Here's how the part is built. I have some questions about the finished solid (model axes, mm). A direction names the side the tool comes from. Coordinates: 2 decimals unless noted, no trailing zeros. Loops run counter-clockwise (first coordinate to the right, second up) from the corner with the lowest first, then second, coordinate; pieces in that order, holes last.
from build123d import *

# Parameters (mm, degrees)
CYLINDER098_R          = 1.8
CYLINDER098_DEPTH      = 5
ARRAY001_X_COUNT       = 2
ARRAY001_X_PITCH       = 31
ARRAY001_Y_COUNT       = 2
ARRAY001_Y_PITCH       = 31
CYLINDER_R             = 2.2
CYLINDER_DEPTH         = 20
ARRAY_X_COUNT          = 2
ARRAY_X_PITCH          = 30
ARRAY_Y_COUNT          = 2
ARRAY_Y_PITCH          = 20
ARRAY_PLACEMENT_ANGLE  = 90
CYLINDER097_R          = 11.5
CYLINDER097_DEPTH      = 5
BOX006_W               = 53
BOX006_H               = 5
BOX006_DEPTH           = 30
BOX005_W               = 53
BOX005_H               = 53
BOX005_DEPTH           = 5
FILLET001_R            = 10
PAD001_DEPTH           = 5
ARRAY002_X_COUNT       = 2
ARRAY002_X_PITCH       = 48
CUT004_ROLL_ANGLE      = 90
CUT004_PLACEMENT_ANGLE = -90


with BuildPart() as stepper_bolt_hole_array:
    # Cylinder098 → Cylinder098 (new body)
    with BuildSketch(Plane.XY):
        Circle(CYLINDER098_R)
    extrude(amount=CYLINDER098_DEPTH)

    # Array001 X: stepper bolt hole array ×2


with BuildPart() as stepper_bolt_hole_array_1:
    add(stepper_bolt_hole_array.part)
    with Locations(*[(i * ARRAY001_X_PITCH, 0, 0) for i in range(1, ARRAY001_X_COUNT)]):
        add(stepper_bolt_hole_array.part)

    # Array001 Y: stepper bolt hole array ×2


with BuildPart() as stepper_bolt_hole_array_2:
    add(stepper_bolt_hole_array_1.part)
    with Locations(*[(0, i * ARRAY001_Y_PITCH, 0) for i in range(1, ARRAY001_Y_COUNT)]):
        add(stepper_bolt_hole_array_1.part)


with BuildPart() as stepper_bolt_hole_array_3:
    # Array001 placement: moved
    add(stepper_bolt_hole_array_2.part.moved(Location((-15.5, -15.5, 0))))


with BuildPart() as insert_hole_array:
    # Cylinder → Cylinder (new body)
    with BuildSketch(Plane.XY.offset(-3)):
        Circle(CYLINDER_R)
    extrude(amount=CYLINDER_DEPTH)

    # Array X: insert hole array ×2


with BuildPart() as insert_hole_array_1:
    add(insert_hole_array.part)
    with Locations(*[(i * ARRAY_X_PITCH, 0, 0) for i in range(1, ARRAY_X_COUNT)]):
        add(insert_hole_array.part)

    # Array Y: insert hole array ×2


with BuildPart() as insert_hole_array_2:
    add(insert_hole_array_1.part)
    with Locations(*[(0, i * ARRAY_Y_PITCH, 0) for i in range(1, ARRAY_Y_COUNT)]):
        add(insert_hole_array_1.part)


with BuildPart() as insert_hole_array_3:
    # Array placement: moved
    add(insert_hole_array_2.part.moved(Location((-15, -20.5, 10))).rotate(Axis((-15, -20.5, 10), (1, 0, 0)), ARRAY_PLACEMENT_ANGLE))


with BuildPart() as stepper_mount_holes:
    # Cylinder097 → Cylinder097 (new body)
    with BuildSketch(Plane.XY):
        Circle(CYLINDER097_R)
    extrude(amount=CYLINDER097_DEPTH)

    # Fusion006: union stepper bolt hole array, insert hole array
    add(stepper_bolt_hole_array_3.part)
    add(insert_hole_array_3.part)


with BuildPart() as stepper_mount_bottom:
    # Box006 → Box006 (new body)
    with BuildSketch(Plane(origin=(-26.5, -26.5, 5), x_dir=(1, 0, 0), z_dir=(0, 0, 1))):
        with Locations((26.5, 2.5)):
            Rectangle(BOX006_W, BOX006_H)
    extrude(amount=BOX006_DEPTH)


with BuildPart() as stepper_mount_cube_fillet:
    # Box005 → Box005 (new body)
    with BuildSketch(Plane(origin=(-26.5, -26.5, 0), x_dir=(1, 0, 0), z_dir=(0, 0, 1))):
        with Locations((26.5, 26.5)):
            Rectangle(BOX005_W, BOX005_H)
    extrude(amount=BOX005_DEPTH)

    # Fillet001
    fillet001_edges = [stepper_mount_cube_fillet.edges().sort_by_distance(p)[0] for p in [
        (-26.5, 26.5, 2.5),
        (26.5, 26.5, 2.5),
    ]]
    fillet(fillet001_edges, radius=FILLET001_R)


with BuildPart() as stepper_mount_cut:
    # Sketch001 → Pad001 (new body)
    with BuildSketch(Plane.YZ):
        Polygon((-26.5, 5), (-3.224222, 5), (-26.5, 35), align=None)
    extrude(amount=PAD001_DEPTH)

    # Array002 X: stepper mount cut ×2


with BuildPart() as stepper_mount_cut_1:
    add(stepper_mount_cut.part)
    with Locations(*[(i * ARRAY002_X_PITCH, 0, 0) for i in range(1, ARRAY002_X_COUNT)]):
        add(stepper_mount_cut.part)


with BuildPart() as stepper_mount_cut_2:
    # Array002 placement: moved
    add(stepper_mount_cut_1.part.moved(Location((-26.5, 0, 0))))

    # Fusion007: union stepper mount bottom, stepper mount cube fillet
    add(stepper_mount_bottom.part)
    add(stepper_mount_cube_fillet.part)

    # Cut004: cut stepper mount holes
    add(stepper_mount_holes.part, mode=Mode.SUBTRACT)


with BuildPart() as stepper_mount_cut_3:
    # Cut004 roll: moved
    add(stepper_mount_cut_2.part.rotate(Axis((0, 0, 0), (1, 0, 0)), CUT004_ROLL_ANGLE))


with BuildPart() as stepper_mount_cut_4:
    # Cut004 placement: moved
    add(stepper_mount_cut_3.part.moved(Location((0, 0, 21.5))).rotate(Axis((0, 0, 21.5), (0, 0, 1)), CUT004_PLACEMENT_ANGLE))


solid = stepper_mount_cut_4.part
Q1. Will these pins go through, and if not, where does the flat tip stop? P1, Ø20.5, axis at y = 0, z = 21.5, coming from the -X side; P2, Ø2, axis at x = -29.5, y = -13.5, coming from the +Z side; P3, Ø8, axis at y = -3, z = 42.5, coming from the -X side.
Q2. We'd pull the mould along X, two halves only. Please class faces 1 (the cylindrical face through (-10.66, -17.1, -2.46)), 2 (the flat face through (-2, 0, 48)), 3 (the flat face through (-35, 0, -2)): pulls with the +X half, pulls with the -X half, needs draft (parallel to the pull), parting line crosses it, or undercut.
Q3. Suppose I cut it at B-B on y = 4. Write out the boundary of the cut face in (x, z).
Q4. Suppose I cut it at D-D on y = 15.5. Write out the boundary of the cut face in (x, z), and give its area (3 significant figures).
Q5. Suppose I cut it at C-C on z = 26.5. Write out the boundary of the cut face in (x, y).
Q6. Suppose I cut it at A-A on x = -3.5. Write out the boundary of the cut face in (y, z).
Q7. For faces 4 (the flat face through (-12, 21.5, 5)), 5 (the flat face through (-17, 0, -5)), which set-ups out of +Z, -Z, +X, -X, +Y, -Y let a thin tool reach every point of the face, with its end or its side?
Q8. Please list where these lines run through material, in increasing order: probe 1 along X at (y, z) = (-15, -3.9); probe 2 along Z at (x, y) = (-2.5, 15.5); probe 3 along Z at (x, y) = (-1.7, 0).
Check values:
1. P1: passes through
1. P2: stops at z = 0
1. P3: stops at x = -5
2. face 1: undercut
2. face 2: needs draft
2. face 3: pulls with the -X half
3. outline: (-35, -5) - (0, -5) - (0, 10.72) - (-5, 10.72) - (-5, 0) - (-35, 0) - close; (-5, 32.28) - (0, 32.28) - (0, 48) - (-5, 48) - close
4. outline: (-35, -5) - (-32.14, -5) - (-32.14, 0) - (-35, 0) - close; (-27.86, -5) - (-12.14, -5) - (-12.14, 0) - (-27.86, 0) - close; (-7.86, -5) - (0, -5) - (0, 4.2) - (-5, 4.2) - (-5, 0) - (-7.86, 0) - close; (-5, 7.8) - (0, 7.8) - (0, 35.2) - (-5, 35.2) - close; (-5, 38.8) - (0, 38.8) - (0, 48) - (-5, 48) - close
4. area: 336 mm2
5. outline: (-5, -26.5) - (0, -26.5) - (0, -10.36) - (-5, -10.36) - close; (-5, 10.36) - (0, 10.36) - (0, 26.5) - (-5, 26.5) - close
6. outline: (-26.5, -5) - (26.5, -5) - (26.5, 38) arc R10 ccw to (16.5, 48) - (-16.5, 48) arc R10 ccw to (-26.5, 38) - close; hole circle Ø3.6 at (-15.5, 6); hole circle Ø3.6 at (-15.5, 37); hole circle Ø23 at (0, 21.5); hole circle Ø3.6 at (15.5, 6); hole circle Ø3.6 at (15.5, 37)
7. face 4: +Z, -X
7. face 5: -Z, +X, -X, +Y, -Y
8. probe 1: x = -35 to -32.2, -27.8 to -12.2, -7.8 to 0
8. probe 2: z = -5 to 4.2, 7.8 to 35.2, 38.8 to 48
8. probe 3: z = -5 to 10, 33 to 48
